Part model, mm, in its own coordinate system. A direction names the side the tool comes from. Round coordinates to 2 decimals unless told otherwise and drop trailing zeros. Loops run counter-clockwise (first coordinate to the right, second up) from the corner with the lowest first, then second, coordinate; pieces in that order, holes last. Notation, with made-up numbers: (69, 57.25) - (84, 57.25) arc R22 ccw to (84, 75.25) - close; hole circle Ø8 at (69.5, 23.5). An arc over 180 degrees is marked (long way). Put each result on its own line as item: value.
from build123d import *

# Parameters (mm, degrees)
F0_W      = 120
F0_H      = 50
F1_DEPTH  = 60
F2_W      = 30
F2_H      = 40
F2_W_2    = 20
F2_H_2    = 30
F3_DEPTH  = 25
F5_DEPTH  = 15
F7_SIZE   = 20
F8_R      = 20
F9_DEPTH  = 10
F10_R     = 4
F11_DEPTH = 20
F6_W      = 120
F6_H      = 60
F12_DEPTH = 20
F13_R     = 6
F14_DEPTH = 20
F15_R     = 3
F16_R     = 3


with BuildPart() as f1:
    # F0 (on Front) → F1 (new body)
    with BuildSketch(Plane.XZ):
        with Locations((-60, 25)):
            Rectangle(F0_W, F0_H)
    extrude(amount=F1_DEPTH)

    # F2 (on face) → F3 (cut)
    with BuildSketch(Plane.XY.offset(50)):
        with Locations((-97, -30)):
            Rectangle(F2_W, F2_H)
        with Locations((-97, -30)):
            Rectangle(F2_W_2, F2_H_2, mode=Mode.SUBTRACT)
    extrude(amount=-F3_DEPTH, mode=Mode.SUBTRACT)

    # F4 (on face) → F5 (cut)
    with BuildSketch(Plane.XY.offset(50)):
        with BuildLine():
            ThreePointArc((-97, -21), (-99.828427, -22.171573), (-101, -25))
            Line((-101, -25), (-101, -35))
            ThreePointArc((-101, -35), (-99.828427, -37.828427), (-97, -39))
            ThreePointArc((-97, -39), (-94.171573, -37.828427), (-93, -35))
            Line((-93, -35), (-93, -25))
            ThreePointArc((-93, -25), (-94.171573, -22.171573), (-97, -21))
        make_face()
    extrude(amount=-F5_DEPTH, mode=Mode.SUBTRACT)

    # F7
    f7_edges = [f1.edges().sort_by_distance(p)[0] for p in [
        (0, -30, 50),
    ]]
    chamfer(f7_edges, length=F7_SIZE)

    # F8 (on face) → F9 (cut)
    with BuildSketch(Plane.XY.offset(50)):
        with Locations((-52, -30)):
            Circle(F8_R)
    extrude(amount=-F9_DEPTH, mode=Mode.SUBTRACT)

    # F10 (on face) → F11 (cut)
    with BuildSketch(Plane.XY.offset(40)):
        with Locations((-52.059621, -17)):
            Circle(F10_R)
        with Locations((-63.288141, -23.551633)):
            Circle(F10_R)
        with Locations((-63.22852, -36.551633)):
            Circle(F10_R)
        with Locations((-51.940379, -43)):
            Circle(F10_R)
        with Locations((-40.711859, -36.448367)):
            Circle(F10_R)
        with Locations((-40.77148, -23.448367)):
            Circle(F10_R)
    extrude(amount=-F11_DEPTH, mode=Mode.SUBTRACT)

    # F6 (on face) → F12 (cut)
    with BuildSketch(Plane(origin=(0, 0, 0), x_dir=(1, 0, 0), z_dir=(0, 0, -1))):
        with Locations((-60, 30)):
            Rectangle(F6_W, F6_H)
    extrude(amount=-F12_DEPTH, mode=Mode.SUBTRACT)

    # F13 (on face) → F14 (cut)
    with BuildSketch(Plane.XY.offset(40)):
        with Locations((-52, -30)):
            Circle(F13_R)
    extrude(amount=-F14_DEPTH, mode=Mode.SUBTRACT)

    # F15
    f15_edges = [f1.edges().sort_by_distance(p)[0] for p in [
        (-120, -60, 35),
    ]]
    fillet(f15_edges, radius=F15_R)

    # F16
    f16_edges = [f1.edges().sort_by_distance(p)[0] for p in [
        (-120, 0, 35),
    ]]
    fillet(f16_edges, radius=F16_R)


solid = f1.part
1. Tool access for faces 1 (the flat face through (-97, -10, 38)), 2 (the flat face through (-81.8, -29.6, 50)): list every direction of +Z, -Z, +X, -X, +Y, -Y with a clear straight run to the whole face (end or side of a thin tool).
A:
face 1: +Z
face 2: +Z, +X, -X, +Y, -Y
2. Probe line 1 along Y through (x, z) = (-105, 44.75); line 2 along X through (y, z) = (-25, 22.25); line 3 along X through (y, z) = (-41.5, 25.5). List the from-to ranges inside material, lowest first. Write a range as [from, to].
A:
line 1: y = [-60, -50], [-45, -15], [-10, 0]
line 2: x = [-120, -67.02], [-59.56, -55.32], [-48.68, -44.46], [-37.08, 0]
line 3: x = [-120, -112], [-107, -87], [-82, -55.65], [-48.23, 0]
3. Band-saw the part on B-B (y = -30). List the corners of the cut face in (x, z), plus the area to 3 significant figures.
A:
outline: (-120, 20) - (-58, 20) - (-58, 40) - (-72, 40) - (-72, 50) - (-82, 50) - (-82, 25) - (-87, 25) - (-87, 50) - (-93, 50) - (-93, 35) - (-101, 35) - (-101, 50) - (-107, 50) - (-107, 25) - (-112, 25) - (-112, 50) - (-120, 50) - close; (-46, 20) - (0, 20) - (0, 30) - (-20, 50) - (-32, 50) - (-32, 40) - (-46, 40) - close
area: 2,390 mm²
4. Pin check, flat tips, straight feed: P1, Ø5, axis at x = -63.29, y = -23.55, coming from the -Z side; P2, Ø9, axis at x = -40.71, y = -36.45, coming from the +Z side. Stop position of each tip, or through.
A:
P1: passes through
P2: stops at z = 40
5. Band-saw the part on A-A (z = 41.25). List the corners of the cut face in (x, y), plus the area to 3 significant figures.
A:
outline: (-120, -57) arc R3 ccw to (-117, -60) - (-11.25, -60) - (-11.25, 0) - (-117, 0) arc R3 ccw to (-120, -3) - close; (-107, -45) - (-87, -45) - (-87, -15) - (-107, -15) - close; hole (-112, -50) - (-82, -50) - (-82, -10) - (-112, -10) - close; hole (-101, -35) arc R4 ccw to (-93, -35) - (-93, -25) arc R4 ccw to (-101, -25) - close; hole circle Ø40 at (-52, -30)
area: 4,530 mm²
6. Two-plate mould, pull along Y, no slides. Class faces 3 (the cylindrical face through (-119.14, -0.9, 35.21)), 4 (the flat face through (-93, -30, 43)), 5 (the flat face through (-10, -30, 40)): pulls with the +Y half, pulls with the -Y half, needs draft (parallel to the pull), parting line crosses it, or undercut.
A:
face 3: pulls with the +Y half
face 4: undercut
face 5: needs draft
7. Band-saw the part on C-C (x = -51.5). List the corners of the cut face in (y, z).
A:
outline: (-60, 20) - (-46.98, 20) - (-46.98, 40) - (-49.99, 40) - (-49.99, 50) - (-60, 50) - close; (-39.02, 20) - (-35.98, 20) - (-35.98, 40) - (-39.02, 40) - close; (-24.02, 20) - (-20.96, 20) - (-20.96, 40) - (-24.02, 40) - close; (-13.04, 20) - (0, 20) - (0, 50) - (-10.01, 50) - (-10.01, 40) - (-13.04, 40) - close
8. Band-saw the part on D-D (y = -17). List the corners of the cut face in (x, z), plus the area to 3 significant figures.
A:
outline: (-120, 20) - (-56.06, 20) - (-56.06, 40) - (-67.2, 40) - (-67.2, 50) - (-82, 50) - (-82, 25) - (-87, 25) - (-87, 50) - (-107, 50) - (-107, 25) - (-112, 25) - (-112, 50) - (-120, 50) - close; (-48.06, 20) - (0, 20) - (0, 30) - (-20, 50) - (-36.8, 50) - (-36.8, 40) - (-48.06, 40) - close
area: 2,690 mm²
